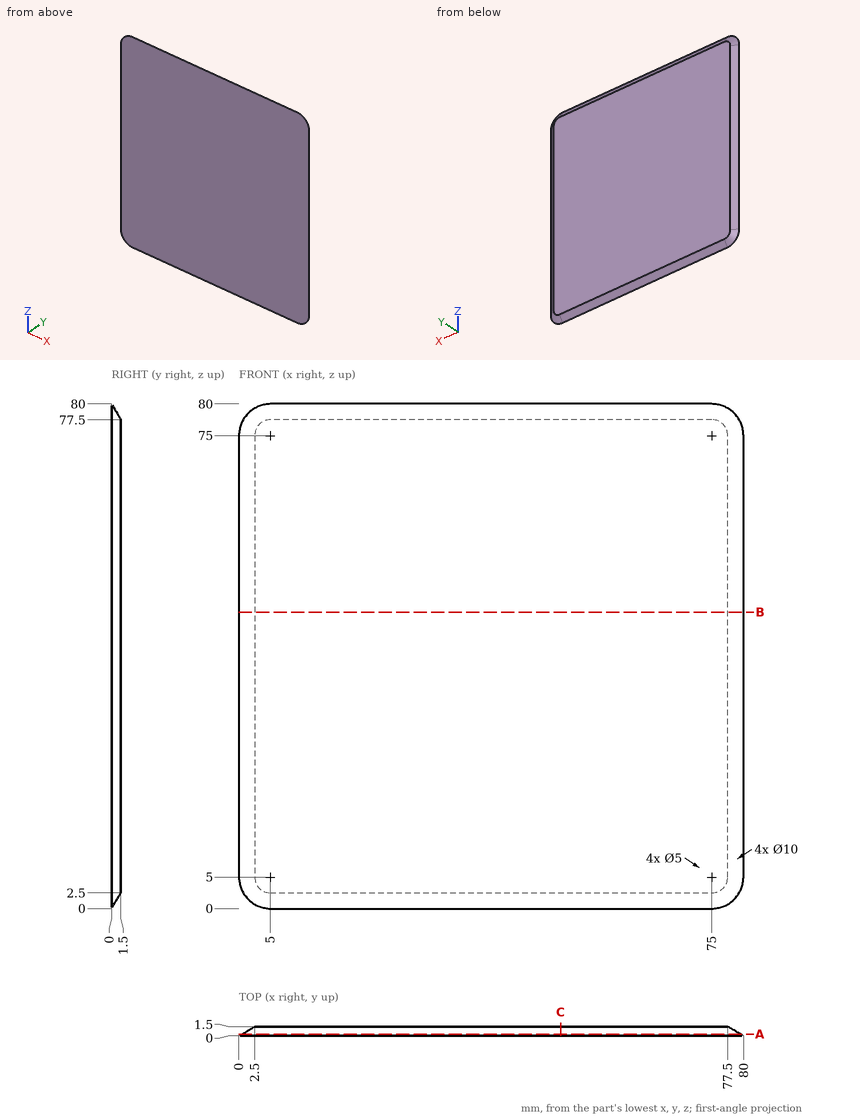
For this review, use the dimensioned drawing (mm, ordinates from the lowest corner) and the shaded views. Coordinates: 2 decimals unless noted, no trailing zeros. Order: outer loops, then holes, each group sorted by start corner. A loop starts at its lowest first (then second) coordinate and runs counter-clockwise, first axis right, second up. Notation, with made-up numbers: (23.5, 80) - (44.5, 80) arc R18 cw to (44.5, 92) - close; hole circle Ø10 at (52.5, 40). An arc over 180 degrees is marked (long way). Answer in a Markdown table with one row per item.
(1) Consider section A-A on y = 0.3. State the section outline as (x, z) points.
Checked values:
| item | result |
|---|---|
| outline | (0.5, 5) arc R4.5 ccw to (5, 0.5) - (75, 0.5) arc R4.5 ccw to (79.5, 5) - (79.5, 75) arc R4.5 ccw to (75, 79.5) - (5, 79.5) arc R4.5 ccw to (0.5, 75) - close |
(2) Wall thickness on line 1 along X through (y, z) = (0.55, 44); line 2 along Z through (x, y) = (66, 0.3); line 3 along Z through (x, y) = (59.5, 0.95): over which ranges is each line inside the solid? List them lowest first. Write a range as from..to.
Checked values:
| item | result |
|---|---|
| line 1 | 0.92..79.08 |
| line 2 | 0.5..79.5 |
| line 3 | 1.58..78.42 |
(3) Consider section C-C on x = 51. State the section outline as (y, z) points.
Checked values:
| item | result |
|---|---|
| outline | (0, 0) - (1.5, 2.5) - (1.5, 77.5) - (0, 80) - close |
(4) Consider section B-B on z = 47. State the section outline as (x, y) points.
Checked values:
| item | result |
|---|---|
| outline | (0, 0) - (80, 0) - (77.5, 1.5) - (2.5, 1.5) - close |
